Part model, mm, in its own coordinate system. A direction names the side the tool comes from. Coordinates: 2 decimals unless noted, no trailing zeros. Write each loop counter-clockwise with the first axis right and the second up, starting at its lowest first coordinate (ties: lowest second). Pieces come first, ordered by that corner, then holes. Notation, with made-up numbers: (73.5, 72) - (127.5, 72) arc R8 cw to (127.5, 83) - close; hole circle Ø10 at (0.5, 31). An arc over 180 degrees is marked (long way). Use a Markdown table: item, result.
```python
from build123d import *

# Parameters (mm, degrees)
SKETCH2_R = 2.032


with BuildPart() as part:
    # Base-Sweep: sweep along a path in Sketch1
    with BuildLine(Plane.XY) as base_sweep_path:
        Line((-56.515, 0), (-49.1998, 0))
        ThreePointArc((-49.1998, 0), (-45.841184211, 1.391184211), (-44.45, 4.7498))
        Line((-44.45, 4.7498), (-44.45, 46.0502))
        ThreePointArc((-44.45, 46.0502), (-43.058815789, 49.408815789), (-39.7002, 50.8))
        Line((-39.7002, 50.8), (39.7002, 50.8))
        ThreePointArc((39.7002, 50.8), (43.058815789, 49.408815789), (44.45, 46.0502))
        Line((44.45, 46.0502), (44.45, 4.7498))
        ThreePointArc((44.45, 4.7498), (45.841184211, 1.391184211), (49.1998, 0))
        Line((49.1998, 0), (56.515, 0))
    # Sketch2 → Base-Sweep (sweep)
    with BuildSketch(Plane(origin=(56.515, 0, 0), x_dir=(0, 0, -1), z_dir=(1, 0, 0))):
        Circle(SKETCH2_R)
    sweep(path=base_sweep_path.line)


solid = part.part
```
Item 1: Drill centre lines: probe 1 along X at (y, z) = (43.5, 1.05); probe 2 along X at (y, z) = (20, -1.6); probe 3 along Y at (x, z) = (-7.5, 0.2). Where is each one in solid material? Low to high.
From the geometry:
| item | result |
|---|---|
| probe 1 | -46.19 to -42.71, 42.71 to 46.19 |
| probe 2 | -45.7 to -43.2, 43.2 to 45.7 |
| probe 3 | 48.78 to 52.82 |
Item 2: Band-saw the part on C-C, the plane x = 18. Give the cut face in (y, z).
From the geometry:
| item | result |
|---|---|
| outline | circle Ø4.06 at (50.8, 0) |
Item 3: Band-saw the part on A-A, the plane z = 0. Give the cut face in (x, y) (3 decimals).
From the geometry:
| item | result |
|---|---|
| outline | (-56.515, -2.032) - (-49.2, -2.032) arc R6.782 ccw to (-42.418, 4.75) - (-42.418, 46.05) arc R2.718 cw to (-39.7, 48.768) - (39.7, 48.768) arc R2.718 cw to (42.418, 46.05) - (42.418, 4.75) arc R6.782 ccw to (49.2, -2.032) - (56.515, -2.032) - (56.515, 2.032) - (49.2, 2.032) arc R2.718 cw to (46.482, 4.75) - (46.482, 46.05) arc R6.782 ccw to (39.7, 52.832) - (-39.7, 52.832) arc R6.782 ccw to (-46.482, 46.05) - (-46.482, 4.75) arc R2.718 cw to (-49.2, 2.032) - (-56.515, 2.032) - close |
Item 4: Two-plate mould, pull along X, no slides. Class faces 4 (the face through (56.515, 0, 0)), 5 (the face through (52.909, -1.984, 0.44)), 6 (the face through (42.466, 25.111, 0.44)): pulls with the +X half, pulls with the -X half, needs draft (parallel to the pull), parting line crosses it, or undercut.
From the geometry:
| item | result |
|---|---|
| face 4 | pulls with the +X half |
| face 5 | needs draft |
| face 6 | undercut |
Item 5: Band-saw the part on B-B, the plane y = 20. Give the cut face in (x, z), then the cut area to 3 significant figures.
From the geometry:
| item | result |
|---|---|
| outline | circle Ø4.06 at (-44.45, 0); circle Ø4.06 at (44.45, 0) |
| area | 25.9 mm^2 |
Item 6: Which spindle directions (+Z, -Z, +X, -X, +Y, -Y) get a long thin tool onto all of the face, cutting with end or side? Do faces 1 (the face through (-56.515, 0, 0)), 2 (the face through (-42.466, 25.689, 0.44)), 3 (the face through (-52.806, -1.984, 0.44)). Say none if no direction does.
From the geometry:
| item | result |
|---|---|
| face 1 | +Z, -Z, -X, +Y, -Y |
| face 2 | none |
| face 3 | -X |
Item 7: Drop flat-ended pins along their axis: P1, Ø2, axis at x = 41.5, y = 47.5, coming from the +Z side (3 decimals); P2, Ø1, axis at x = -37.5, z = 0.5, coming from the +Y side; P3, Ø2, axis at x = 5, z = -1.5, coming from the -Y side. Give the stop position or say it passes through.
From the geometry:
| item | result |
|---|---|
| P1 | z = 1.435 |
| P2 | y = 52.83 |
| P3 | y = 48.83 |
